Autodesk Inventor part; units mm, degrees
ref_plane "YZ Plane" through (0, 0, 0) normal (1, 0, 0) x (0, 1, 0)
ref_plane "XZ Plane" through (0, 0, 0) normal (0, 1, 0) x (-1, 0, 0)
ref_plane "XY Plane" through (0, 0, 0) normal (0, 0, 1) x (1, 0, 0)
sketch "Sketch1" plane through (0, 0, 0) normal (0, 0, 1) x (1, 0, 0)
  line L0 (6.35, 28.575) -> (25.4, 28.575)
  line L1 (6.35, 31.75) -> (25.4, 31.75)
  line L2 (25.4, 0) -> (6.35, 0)
  arc A0 (0, 6.35) -> (6.35, 0) centre (6.35, 6.35) ccw
  line L3 (0, 6.35) -> (0, 25.4)
  arc A1 (6.35, 31.75) -> (0, 25.4) centre (6.35, 25.4) ccw
  line L4 (6.35, 31.75) -> (25.4, 31.75)
  line L5 (25.4, 28.575) -> (6.35, 28.575)
  arc A2 (6.35, 28.575) -> (3.175, 25.4) centre (6.35, 25.4) ccw
  line L6 (3.175, 25.4) -> (3.175, 6.35)
  arc A3 (3.175, 6.35) -> (6.35, 3.175) centre (6.35, 6.35) ccw
  line L7 (6.35, 3.175) -> (25.4, 3.175)
  line L8 (28.575, 3.175) -> (28.575, 0)
  line L9 (25.4, 31.75) -> (28.575, 31.75)
  line L10 (28.575, 28.575) -> (25.4, 28.575)
  line L11 (28.575, 31.75) -> (28.575, 28.575)
  line L12 (28.575, 0) -> (25.4, 0)
  line L13 (28.575, 3.175) -> (28.575, 0)
  line L14 (25.4, 3.175) -> (28.575, 3.175)
  point P0 (0, 0)
extrude "Extrusion1" add sketch "Sketch1" against normal blind 762
chamfer "Chamfer1" distance 3.175 angle 45 4 edges at (28.575, 30.1625, 0) (28.575, 1.5875, 0) (28.575, 30.1625, -762) (28.575, 1.5875, -762)
sketch "Sketch2" plane through (6.35, 31.75, 0) normal (0, 1, 0) x (1, 0, 0)
  line L0 (19.05, 0) -> (0, 0)
  line L1 (22.225, 3.175) -> (22.225, 758.825)
  point P0 (-6.35, 0)
  point P1 (9.525, 12.7)
  dimension "d5" = 12.7
  dimension "d6" = 12.7
hole "Hole1" at (15.875, 31.75, -12.7) direction (0, -1, 0) diameter 6.7056 end through all
pattern_linear "Rectangular Pattern1" count 30 spacing 25.4 along (0, 0, -1) of "Hole1"
sketch "Sketch3" plane through (0, 6.35, 0) normal (-1, 0, 0) x (0, 0, 1)
  line L0 (0, 19.05) -> (-762, 19.05)
  line L1 (-762, 19.05) -> (-762, 0)
  line L2 (0, 0) -> (-762, 0)
  line L3 (0, 0) -> (0, 19.05)
  circle A0 centre (-701.3194, 9.525) radius 4.8006
  circle A1 centre (-111.4298, 9.525) radius 4.8006
  circle A2 centre (-189.2808, 9.525) radius 3.683
  circle A3 centre (-278.1808, 9.525) radius 3.683
  circle A4 centre (-483.7938, 9.525) radius 3.683
  circle A5 centre (-572.6938, 9.525) radius 3.683
  circle A6 centre (-471.1065, 9.525) radius 3.683
  circle A7 centre (-585.4065, 9.525) radius 3.683
  circle A8 centre (-290.8935, 9.525) radius 3.683
  circle A9 centre (-176.5935, 9.525) radius 3.683
  circle A10 centre (-553.7327, 9.525) radius 4.8006
  circle A11 centre (-528.3327, 9.525) radius 4.8006
  circle A12 centre (-502.9327, 9.525) radius 4.8006
  circle A13 centre (-259.0673, 9.525) radius 4.8006
  circle A14 centre (-233.6673, 9.525) radius 4.8006
  circle A15 centre (-208.2673, 9.525) radius 4.8006
  circle A16 centre (-609.6, 9.525) radius 1.5875
  circle A17 centre (-152.4, 9.525) radius 1.5875
  circle A18 centre (-381, 5.969) radius 4.8006
  circle A19 centre (-86.0298, 9.525) radius 4.8006
  circle A20 centre (-675.9194, 9.525) radius 4.8006
  circle A21 centre (-650.5194, 9.525) radius 4.8006
  circle A22 centre (-60.6298, 9.525) radius 4.8006
  point P0 (0, -6.35)
  point P1 (-762, -6.35)
extrude "Extrusion2" cut sketch "Sketch3" against normal up to next contours A0 | A1 | A2 | A3 | A4 | A5 | A6 | A7 | A8 | A9 | A10 | A11 | A12 | A13 | A14 | A15 | A16 | A17 | A18 | A19 | A20 | A21 | A22
sketch "Sketch4" plane through (6.35, 31.75, 0) normal (0, 1, 0) x (1, 0, 0)
  line L0 (-21.9023, 506.5738) -> (102.4291, 506.5738)
  line L1 (102.4291, 506.5738) -> (102.4291, -101.978)
  line L2 (102.4291, -101.978) -> (-21.9023, -101.978)
  line L3 (-21.9023, -101.978) -> (-21.9023, 506.5738)
  point P0 (-6.35, 0)
extrude "Extrusion3" cut sketch "Sketch4" against normal blind 50.8
sketch "Sketch5" plane through (6.35, 31.75, -762) normal (0, 1, 0) x (1, 0, 0)
  line L0 (0, -255.4262) -> (0, 0)
  line L1 (0, 0) -> (22.225, -22.2443)
  line L2 (22.225, -255.4262) -> (22.225, -3.175)
  line L3 (0, 0) -> (19.05, 0)
  line L4 (0, 0) -> (22.225, 0)
  line L5 (22.225, 0) -> (22.225, -22.2443)
  point P0 (-6.35, -762)
extrude "Extrusion4" cut sketch "Sketch5" against normal blind 76.2
properties part number "am-2222" material "Aluminum 6061"
Here's how the part is built. I have some questions about the finished solid (model axes, mm). Give positions to 0.01 mm unless a question says otherwise; leave off trailing zeros. Write each loop counter-clockwise with the first axis right and the second up, starting at its lowest first coordinate (ties: lowest second). Pieces come first, ordered by that corner, then holes. Notation, with made-up numbers: (32.5, 14.5) -> (75.5, 14.5) arc R18 cw to (75.5, 24.5) -> close; hole circle Ø11 at (56.25, -32). An arc over 180 degrees is marked (long way). Use one line per item in the form item = value. Start each with the question number.
1. Imagine slicing it at A-A on z = -723.9. List the corners of the cut face in (x, y) for me (3 decimals), plus the area to 3 significant figures.
2. Imagine slicing it at D-D on y = 8.5. List the corners of the cut face in (x, z) for me (3 decimals).
3. If I drill on L1, parallel to Y at x = 12.5, z = -697.5 (3 decimals); L2, parallel to X at y = 29.5, z = -621.5 (3 decimals); L3, parallel to X at y = 29, z = -675.5 (3 decimals), over which ranges is the centre line in solid material (lowest first)?
4. Thinking about a two-plate mould opening in X: for faces 1 (the face through (23.833, 1.61, -744.501)), 2 (the face through (14.87, 1.57, -517.5)), 3 (the face through (17, 31.75, -632)), which applies, +X half, -X half, draft (parallel to the pull), parting line (faces both ways), or undercut?
5. Will this pin go through, and if not, where does the flat tip stop? pin 1 Ø3 at (y, z) = (7.5, -689.5) entering from +X.
6. Imagine slicing it at C-C on z = -571.5. List the corners of the cut face in (x, y) for me (3 decimals).
7. Imagine slicing it at B-B on x = 24.25. List the corners of the cut face in (y, z) for me (3 decimals).
Entries:
q1.outline = (0, 6.35) arc R6.35 ccw to (6.35, 0) -> (12.522, 0) -> (12.522, 3.175) -> (6.35, 3.175) arc R3.175 cw to (3.175, 6.35) -> (3.175, 25.4) arc R3.175 cw to (6.35, 28.575) -> (12.522, 28.575) -> (12.522, 31.75) -> (6.35, 31.75) arc R6.35 ccw to (0, 25.4) -> close; (19.228, 0) -> (28.575, 0) -> (28.575, 3.175) -> (19.228, 3.175) -> close; (19.228, 28.575) -> (28.575, 28.575) -> (28.575, 31.75) -> (19.228, 31.75) -> close
q1.area = 207 mm²
q2.outline = (0, -762) -> (3.175, -762) -> (3.175, -506.574) -> (0, -506.574) -> close
q3.L1 = 0 to 3.175, 28.575 to 31.75
q3.L2 = 1.501 to 12.619, 19.131 to 28.575
q3.L3 = 1.119 to 13.534, 18.216 to 28.575
q4.face_1 = +X half
q4.face_2 = undercut
q4.face_3 = draft
q5.pin_1 = 3.19
q6.outline = (0, 6.35) arc R6.35 ccw to (6.35, 0) -> (12.522, 0) -> (12.522, 3.175) -> (6.35, 3.175) arc R3.175 cw to (3.175, 6.35) -> (3.175, 12.391) -> (0, 12.391) -> close; (0, 19.359) -> (3.175, 19.359) -> (3.175, 25.4) arc R3.175 cw to (6.35, 28.575) -> (12.522, 28.575) -> (12.522, 31.75) -> (6.35, 31.75) arc R6.35 ccw to (0, 25.4) -> close; (19.228, 0) -> (28.575, 0) -> (28.575, 3.175) -> (19.228, 3.175) -> close; (19.228, 28.575) -> (28.575, 28.575) -> (28.575, 31.75) -> (19.228, 31.75) -> close
q7.outline = (0, -744.084) -> (3.175, -744.084) -> (3.175, -506.574) -> (0, -506.574) -> close; (28.575, -744.084) -> (31.75, -744.084) -> (31.75, -506.574) -> (28.575, -506.574) -> close
